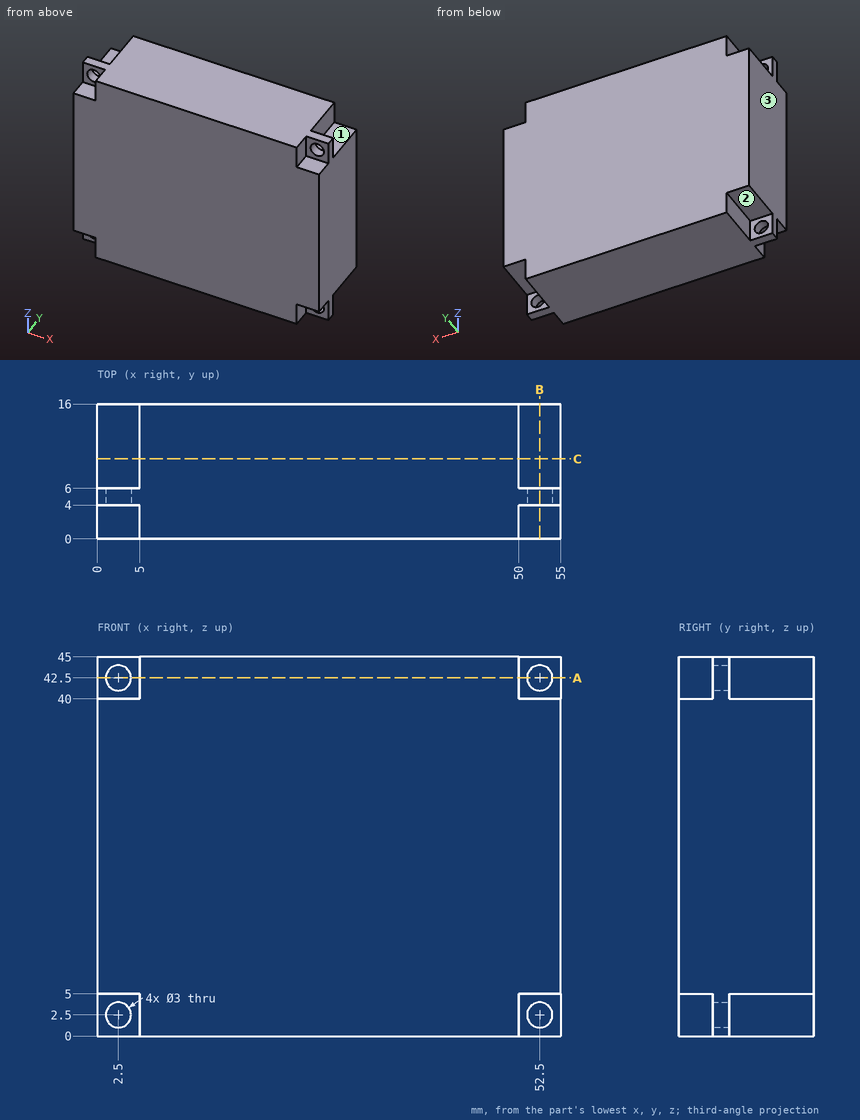
Verification items for this drawing (mm, ordinates from the low corner). A direction names the side the tool comes from. Round coordinates to 2 decimals unless told otherwise and drop trailing zeros. Write each loop counter-clockwise with the first axis right and the second up, starting at its lowest first coordinate (ties: lowest second). Pieces come first, ordered by that corner, then holes. Notation, with made-up numbers: (76, -36) - (117, -36) arc R27 ccw to (117, -20) - close; hole circle Ø7 at (65.5, -28.75). An arc over 180 degrees is marked (long way). Answer as a JSON object with one key per item and string values. Group by question number.
Q1. Section check A-A, the plane z = 42.5. Enter the section's corners in (x, y), plus the area to 3 significant figures.
Q2. Section check B-B, the plane x = 52.5. Enter the section's corners in (y, z).
Q3. Thickness scan on line 1 (X direction, y = 4.5, z = 2.5); line 2 (Z direction, x = 52.5, y = 4.9); line 3 (X direction, y = 12, z = 3.5). Record the ranges inside material, lowest first.
Q4. Section check C-C, the plane y = 9.5. Enter the section's corners in (x, z), plus the area to 4 significant figures.
Q5. Go/stop test with flat-tipped pins: pin 1 Ø3 at (x, y) = (3, 1) entering from +Z; pin 2 Ø1.5 at (y, z) = (13.5, 41.5) entering from +X; pin 3 Ø2 at (y, z) = (2.5, 2) entering from -X. Record where each tip stops, or that it passes through.
Q6. Tool access check on the marked faces 1, 2 and 3. Record the directions out of +Z, -Z, +X, -X, +Y, -Y that give a thin tool (end or side, any length) a straight path to the whole face; none if there is none.
Found:
{
 "1": {"outline": "(0, 4) - (1, 4) - (1, 6) - (0, 6) - close; (4, 4) - (5, 4) - (5, 0) - (50, 0) - (50, 4) - (51, 4) - (51, 6) - (50, 6) - (50, 16) - (5, 16) - (5, 6) - (4, 6) - close; (54, 4) - (55, 4) - (55, 6) - (54, 6) - close", "area": "728 mm^2"},
 "2": {"outline": "(0, 5) - (4, 5) - (4, 4) - (6, 4) - (6, 5) - (16, 5) - (16, 40) - (6, 40) - (6, 41) - (4, 41) - (4, 40) - (0, 40) - close; (4, 0) - (6, 0) - (6, 1) - (4, 1) - close; (4, 44) - (6, 44) - (6, 45) - (4, 45) - close"},
 "3": {"line 1": "x = 0 to 1, 4 to 51, 54 to 55", "line 2": "z = 0 to 1, 4 to 41, 44 to 45", "line 3": "x = 5 to 50"},
 "4": {"outline": "(0, 5) - (5, 5) - (5, 0) - (50, 0) - (50, 5) - (55, 5) - (55, 40) - (50, 40) - (50, 45) - (5, 45) - (5, 40) - (0, 40) - close", "area": "2,375 mm^2"},
 "5": {"pin 1": "stops at z = 40", "pin 2": "stops at x = 50", "pin 3": "stops at x = 5"},
 "6": {"face 1": "+Z, +X, +Y", "face 2": "-Z, -X, +Y", "face 3": "+Z, -Z, -X, +Y, -Y"}
}
